Autodesk Inventor part; units mm, degrees
ref_plane "YZ Plane" through (0, 0, 0) normal (1, 0, 0) x (0, 1, 0)
ref_plane "XZ Plane" through (0, 0, 0) normal (0, 1, 0) x (-1, 0, 0)
ref_plane "XY Plane" through (0, 0, 0) normal (0, 0, 1) x (1, 0, 0)
sketch "Battery Flat" plane through (0, 0, 0) normal (0, 0, 1) x (1, 0, 0)
  line L0 (83.566, 88.9) -> (-83.566, 88.9) construction
  line L1 (-83.566, 88.9) -> (-83.566, -88.9) construction
  line L2 (-83.566, -88.9) -> (83.566, -88.9) construction
  line L3 (83.566, -88.9) -> (83.566, 88.9) construction
  line L4 (83.566, 88.9) -> (-83.566, -88.9) construction
  line L5 (-83.566, 88.9) -> (83.566, -88.9) construction
  line L6 (83.566, -88.9) -> (-83.566, -88.9) construction
  line L7 (-83.566, -88.9) -> (-83.566, 88.9) construction
  line L8 (-83.566, 88.9) -> (83.566, 88.9) construction
  line L9 (83.566, 88.9) -> (83.566, -88.9) construction
  point P0 (0, 0)
  dimension "d39" = 167.132
  dimension "d40" = 177.8
sketch "Circuit Breaker" plane through (0, 0, 0) normal (0, 0, 1) x (1, 0, 0)
  line L0 (4.1103, 47.4016) -> (-23.8297, 47.4016) construction
  line L1 (-23.8297, 47.4016) -> (-23.8297, -9.7484) construction
  line L2 (-23.8297, -9.7484) -> (4.1103, -9.7484) construction
  line L3 (4.1103, -9.7484) -> (4.1103, 47.4016) construction
  line L4 (4.1103, 47.4016) -> (-23.8297, -9.7484) construction
  line L5 (-23.8297, 47.4016) -> (4.1103, -9.7484) construction
  circle A0 centre (-23.8297, -9.7484) radius 3.429
  circle A1 centre (4.1103, 47.4016) radius 3.429
  line L6 (4.1103, -9.7484) -> (-23.8297, -9.7484) construction
  line L7 (-23.8297, -9.7484) -> (-23.8297, 47.4016) construction
  line L8 (-23.8297, 47.4016) -> (4.1103, 47.4016) construction
  line L9 (4.1103, 47.4016) -> (4.1103, -9.7484) construction
  line L10 (14.2703, 55.6566) -> (-33.9897, 55.6566) construction
  line L11 (-33.9897, 55.6566) -> (-33.9897, -18.0034) construction
  line L12 (-33.9897, -18.0034) -> (14.2703, -18.0034) construction
  line L13 (14.2703, -18.0034) -> (14.2703, 55.6566) construction
  line L14 (14.2703, 55.6566) -> (-33.9897, -18.0034) construction
  line L15 (-33.9897, 55.6566) -> (14.2703, -18.0034) construction
  point P0 (0, 0)
  point P1 (-9.8597, 18.8266)
  dimension "d62" = 27.94
  dimension "d63" = 57.15
  dimension "d64" = 6.858
  dimension "d65" = 6.858
  dimension "d66" = 48.26
  dimension "d67" = 73.66
sketch "Sketch1" plane through (0, 0, 0) normal (0, 1, 0) x (-1, 0, 0)
  line L0 (95.25, -95.25) -> (-95.25, -95.25) construction
  line L1 (95.25, -90.4875) -> (-95.25, -90.4875)
  line L2 (-95.25, -100.0125) -> (95.25, -100.0125)
  arc A0 (95.25, -100.0125) -> (95.25, -90.4875) centre (95.25, -95.25) ccw
  arc A1 (-95.25, -90.4875) -> (-95.25, -100.0125) centre (-95.25, -95.25) ccw
  line L3 (95.25, 95.25) -> (-95.25, 95.25) construction
  line L4 (95.25, 100.0125) -> (-95.25, 100.0125)
  line L5 (-95.25, 90.4875) -> (95.25, 90.4875)
  arc A2 (95.25, 90.4875) -> (95.25, 100.0125) centre (95.25, 95.25) ccw
  arc A3 (-95.25, 100.0125) -> (-95.25, 90.4875) centre (-95.25, 95.25) ccw
  line L6 (95.25, -95.25) -> (95.25, 95.25) construction
  line L7 (85.725, -95.25) -> (85.725, 95.25)
  line L8 (104.775, 95.25) -> (104.775, -95.25)
  arc A4 (85.725, -95.25) -> (104.775, -95.25) centre (95.25, -95.25) ccw
  arc A5 (104.775, 95.25) -> (85.725, 95.25) centre (95.25, 95.25) ccw
  line L9 (-95.25, -95.25) -> (-95.25, 95.25) construction
  line L10 (-85.725, -95.25) -> (-85.725, 95.25)
  line L11 (-104.775, 95.25) -> (-104.775, -95.25)
  arc A6 (-104.775, -95.25) -> (-85.725, -95.25) centre (-95.25, -95.25) ccw
  arc A7 (-85.725, 95.25) -> (-104.775, 95.25) centre (-95.25, 95.25) ccw
  circle A8 centre (95.25, -95.25) radius 2.4892
  circle A9 centre (95.25, 95.25) radius 2.4892
  circle A10 centre (57.15, -95.25) radius 2.4892
  circle A11 centre (57.15, 95.25) radius 2.4892
  circle A12 centre (19.05, -95.25) radius 2.4892
  circle A13 centre (19.05, 95.25) radius 2.4892
  circle A14 centre (-19.05, -95.25) radius 2.4892
  circle A15 centre (-19.05, 95.25) radius 2.4892
  circle A16 centre (-57.15, -95.25) radius 2.4892
  circle A17 centre (-57.15, 95.25) radius 2.4892
  circle A18 centre (-95.25, -95.25) radius 2.4892
  circle A19 centre (-95.25, 95.25) radius 2.4892
  circle A20 centre (95.25, 57.15) radius 2.4892
  circle A21 centre (-95.25, 57.15) radius 2.4892
  circle A22 centre (95.25, 19.05) radius 2.4892
  circle A23 centre (-95.25, 19.05) radius 2.4892
  circle A24 centre (95.25, -19.05) radius 2.4892
  circle A25 centre (-95.25, -19.05) radius 2.4892
  circle A26 centre (95.25, -57.15) radius 2.4892
  circle A27 centre (-95.25, -57.15) radius 2.4892
  line L12 (-3.175, 100.0125) -> (-3.175, 150.8125)
  line L13 (-3.175, 150.8125) -> (-79.375, 150.8125)
  line L14 (-79.375, 150.8125) -> (-79.375, 100.0125)
  point P0 (0, 0)
  point P1 (0, 0)
  point P2 (0, -95.25)
  point P3 (0, 95.25)
  point P4 (95.25, 0)
  point P5 (-95.25, 0)
  point P6 (0, 0)
  point P7 (0, 0)
  point P8 (85.725, -90.4875)
  point P9 (-85.725, -90.4875)
  point P10 (-85.725, 90.4875)
  point P11 (85.725, 90.4875)
  point P12 (87.0011, -100.0125)
  point P13 (87.0011, 100.0125)
  point P14 (-87.0011, 100.0125)
  point P15 (-87.0011, -100.0125)
  point P16 (-41.275, 150.8125)
  point P17 (-41.275, 150.8125)
  point P18 (-41.275, 125.4125)
  point P19 (-41.275, 125.4125)
  point P20 (-3.175, 125.4125)
  point P21 (-41.275, 125.4125)
  dimension "d41" = 190.5
  dimension "d42" = 190.5
  dimension "d43" = 9.525
  dimension "d44" = 19.05
  dimension "d45" = 4.9784
  dimension "d48" = 38.1
  dimension "d55" = 38.1
  dimension "d60" = 38.1
  dimension "d68" = 76.2
  dimension "d69" = 50.8
  dimension "d75" = 25.4
extrude "Extrusion1" add sketch "Sketch1" along normal blind 6.35 contours A0 L2 A4 L7 L1 | L1 L7 L5 A2 L4 A5 L8 A4 L2 A0 | L7 A4 L2 A6 L10 L1 | L10 A6 L2 A1 L1 | L1 A1 L2 A6 L11 A7 L4 A3 L5 L10 | L7 A5 L4 A2 L5 | L5 L10 A7 L4 A5 L7 | L5 A3 L4 A7 L10
fillet "Fillet1" radius 50.8 4 edges at (87.0011, 3.175, 100.0125) (-87.0011, 3.175, 100.0125) (-87.0011, 3.175, -100.0125) (87.0011, 3.175, -100.0125)
fillet "Fillet1" radius 3.175 4 edges at (-85.725, 3.175, -90.4875) (85.725, 3.175, -90.4875) (85.725, 3.175, 90.4875) (-85.725, 3.175, 90.4875)
extrude "Extrusion2" [suppressed]
fillet "Fillet2" [suppressed]
sketch "Sketch2" plane through (0, 6.35, 0) normal (0, 1, 0) x (1, 0, 0)
  arc A0 (91.5406, -104.023) -> (71.7571, -100.0125) centre (71.7571, -150.8125) ccw
  arc A1 (91.5406, -104.023) -> (104.775, -95.25) centre (95.25, -95.25) ccw
  line L0 (104.775, -95.25) -> (104.775, 95.25)
  arc A2 (104.775, 95.25) -> (91.5406, 104.023) centre (95.25, 95.25) ccw
  arc A3 (71.7571, 100.0125) -> (91.5406, 104.023) centre (71.7571, 150.8125) ccw
  line L1 (71.7571, 100.0125) -> (-71.7571, 100.0125)
  arc A4 (-91.5406, 104.023) -> (-71.7571, 100.0125) centre (-71.7571, 150.8125) ccw
  arc A5 (-91.5406, 104.023) -> (-104.775, 95.25) centre (-95.25, 95.25) ccw
  line L2 (-104.775, 95.25) -> (-104.775, -95.25)
  arc A6 (-104.775, -95.25) -> (-91.5406, -104.023) centre (-95.25, -95.25) ccw
  arc A7 (-71.7571, -100.0125) -> (-91.5406, -104.023) centre (-71.7571, -150.8125) ccw
  line L3 (-71.7571, -100.0125) -> (71.7571, -100.0125)
  circle A8 centre (-95.25, 95.25) radius 2.4892
  circle A9 centre (-57.15, 95.25) radius 2.4892
  circle A10 centre (-19.05, 95.25) radius 2.4892
  circle A11 centre (19.05, 95.25) radius 2.4892
  circle A12 centre (57.15, 95.25) radius 2.4892
  circle A13 centre (95.25, 95.25) radius 2.4892
  circle A14 centre (-95.25, 57.15) radius 2.4892
  circle A15 centre (-95.25, 19.05) radius 2.4892
  circle A16 centre (-95.25, -19.05) radius 2.4892
  circle A17 centre (-95.25, -57.15) radius 2.4892
  circle A18 centre (-95.25, -95.25) radius 2.4892
  circle A19 centre (-57.15, -95.25) radius 2.4892
  circle A20 centre (-19.05, -95.25) radius 2.4892
  circle A21 centre (19.05, -95.25) radius 2.4892
  circle A22 centre (57.15, -95.25) radius 2.4892
  circle A23 centre (95.25, -95.25) radius 2.4892
  circle A24 centre (95.25, 57.15) radius 2.4892
  circle A25 centre (95.25, -57.15) radius 2.4892
  circle A26 centre (95.25, -19.05) radius 2.4892
  circle A27 centre (95.25, 19.05) radius 2.4892
  line L4 (-82.55, 90.4875) -> (82.55, 90.4875)
  arc A28 (85.725, 87.3125) -> (82.55, 90.4875) centre (82.55, 87.3125) ccw
  line L5 (85.725, 87.3125) -> (85.725, -87.3125)
  arc A29 (82.55, -90.4875) -> (85.725, -87.3125) centre (82.55, -87.3125) ccw
  line L6 (82.55, -90.4875) -> (-82.55, -90.4875)
  arc A30 (-85.725, -87.3125) -> (-82.55, -90.4875) centre (-82.55, -87.3125) ccw
  line L7 (-85.725, -87.3125) -> (-85.725, 87.3125)
  arc A31 (-82.55, 90.4875) -> (-85.725, 87.3125) centre (-82.55, 87.3125) ccw
  arc A32 (7.9375, -144.4625) -> (9.525, -146.05) centre (9.525, -144.4625) ccw
  line L8 (7.9375, -144.4625) -> (7.9375, -106.3625)
  arc A33 (7.9375, -106.3625) -> (-3.175, -95.25) centre (-3.175, -106.3625) ccw
  line L9 (-3.175, -95.25) -> (-71.7571, -95.25)
  arc A34 (-71.7571, -95.25) -> (-93.3953, -99.6365) centre (-71.7571, -150.8125) ccw
  arc A35 (-100.0125, -95.25) -> (-93.3953, -99.6365) centre (-95.25, -95.25) ccw
  line L10 (-100.0125, -95.25) -> (-100.0125, 95.25)
  arc A36 (-93.3953, 99.6365) -> (-100.0125, 95.25) centre (-95.25, 95.25) ccw
  arc A37 (-93.3953, 99.6365) -> (-71.7571, 95.25) centre (-71.7571, 150.8125) ccw
  line L11 (-71.7571, 95.25) -> (71.7571, 95.25)
  arc A38 (71.7571, 95.25) -> (93.3953, 99.6365) centre (71.7571, 150.8125) ccw
  arc A39 (100.0125, 95.25) -> (93.3953, 99.6365) centre (95.25, 95.25) ccw
  line L12 (100.0125, 95.25) -> (100.0125, -95.25)
  arc A40 (93.3953, -99.6365) -> (100.0125, -95.25) centre (95.25, -95.25) ccw
  arc A41 (93.3953, -99.6365) -> (89.217, -98.0646) centre (71.7571, -150.8125) ccw
  arc A42 (89.217, -98.0646) -> (74.6125, -108.6141) centre (85.725, -108.6141) ccw
  line L13 (74.6125, -108.6141) -> (74.6125, -144.4625)
  arc A43 (73.025, -146.05) -> (74.6125, -144.4625) centre (73.025, -144.4625) ccw
  line L14 (73.025, -146.05) -> (9.525, -146.05)
  arc A44 (3.175, -106.3625) -> (-3.175, -100.0125) centre (-3.175, -106.3625) ccw
  line L15 (-3.175, -100.0125) -> (78.6894, -100.0125)
  line L16 (-3.175, -104.775) -> (78.6894, -104.775)
  circle A45 centre (12.7, -111.4425) radius 7.9375
  circle A46 centre (69.85, -139.3825) radius 7.9375
  line L17 (12.7, -111.4425) -> (69.85, -139.3825) construction
  line L18 (11.6541, -113.5818) -> (68.8041, -141.5218)
  line L19 (70.8959, -137.2432) -> (13.7459, -109.3032)
  arc A47 (13.7459, -109.3032) -> (11.6541, -113.5818) centre (12.7, -111.4425) ccw
  arc A48 (68.8041, -141.5218) -> (70.8959, -137.2432) centre (69.85, -139.3825) ccw
  line L20 (2.8572, -144.1945) -> (79.6928, -106.6305) construction
  line L21 (3.9031, -146.3338) -> (80.7387, -108.7697)
  line L22 (78.6469, -104.4912) -> (1.8113, -142.0553)
  arc A49 (1.8113, -142.0553) -> (3.9031, -146.3338) centre (2.8572, -144.1945) ccw
  arc A50 (80.7387, -108.7697) -> (78.6469, -104.4912) centre (79.6928, -106.6305) ccw
  line L23 (41.275, -125.4125) -> (41.275, -104.775) construction
  point P0 (0, 0)
  point P1 (74.6125, -111.7648)
  point P2 (46.6967, -125.4125)
  point P3 (64.0934, -133.9176)
  point P4 (74.6125, -133.0325)
  point P5 (41.275, -122.7619)
  point P6 (74.8457, -106.3496)
  point P7 (75.2967, -104.775)
  point P8 (17.0068, -104.775)
  point P9 (20.5483, -112.6289)
  point P10 (7.9375, -139.0602)
  point P11 (35.8533, -125.4125)
  point P12 (18.4566, -116.9074)
  point P13 (7.9375, -117.7925)
  point P14 (65.5432, -146.05)
  point P15 (62.0017, -138.1961)
  point P16 (41.275, -128.0631)
  point P17 (7.9375, -144.3614)
  dimension "d77" = 4.7625
  dimension "d78" = 15.875
  dimension "d79" = 4.7625
  dimension "d80" = 4.7625
extrude "Extrusion3" [suppressed]
fillet "Fillet3" [suppressed]
equation "\"d42\" = d41"
properties part number "7525-18-800-002 Battery Mount" material "Aluminum 6061"
The model under review builds one solid part; all positions refer to its coordinate system, in mm. A direction names the side the tool comes from. Round coordinates to 2 decimals unless told otherwise and drop trailing zeros. Loops run counter-clockwise (first coordinate to the right, second up) from the corner with the lowest first, then second, coordinate; pieces in that order, holes last. Notation, with made-up numbers: (65, 13) - (97, 13) arc R18 cw to (97, 48) - close; hole circle Ø9 at (44, 31.5). An arc over 180 degrees is marked (long way). Write each question's results on one line, items separated by ' | '. Start each with the question number.
Q1. Take a section at B-B on x = 64.5. Give the boundary of the cut face in (y, z), plus the area to 3 significant figures.
Q2. Tool access review of faces 1 (the cylindrical face through (-81.711, 3.219, 100.997)), 2 (the flat face through (-1, 3, -90.488)), 3 (the cylindrical face through (-100.622, 3.131, -103.116)): name each direction out of +Z, -Z, +X, -X, +Y, -Y from which nothing blocks a thin tool from reaching the whole face with its end or side.
Q3. Insertion check: P1, Ø3, axis at x = -95.25, z = -95.25, coming from the -Y side. The pin has a flat end and moves straight along its axis. Give the tip position at first contact, or say it passes through.
Q4. Take a section at C-C on z = 79. Give the boundary of the cut face in (x, y) (3 decimals).
Q5. Wall thickness on line 1 along X through (y, z) = (2, -57) (3 decimals); line 2 along Z through (x, y) = (-19.05, 5.25); line 3 along Z through (x, y) = (44, 1.5): over which ranges is each line inside the solid? List them lowest first. Write a range as [from, to].
Q6. Take a section at A-A on x = -57.15. Give the boundary of the cut face in (y, z).
Q7. Draft analysis for pull direction X (two halves, no side actions). For faces 4 (the flat face through (-104.775, 3, 1)), 5 (the flat face through (1, 0, -92)), 6 (the flat face through (1, 3, -100.012)), 7 (the cylindrical face through (-97.55, 3.13, 58.1)), state which applies: pulls with the +X half, pulls with the -X half, needs draft (parallel to the pull), parting line crosses it, or undercut.
Q8. Take a section at D-D on x = 95.25. Give the boundary of the cut face in (y, z) (3 decimals).
Data:
1) outline: (0, -100.01) - (6.35, -100.01) - (6.35, -90.49) - (0, -90.49) - close; (0, 90.49) - (6.35, 90.49) - (6.35, 100.01) - (0, 100.01) - close | area: 121 mm²
2) face 1: +Z, +Y, -Y | face 2: +Y, -Y | face 3: -Z, +Y, -Y
3) P1: passes through
4) outline: (-104.775, 0) - (-85.725, 0) - (-85.725, 6.35) - (-104.775, 6.35) - close; (85.725, 0) - (104.775, 0) - (104.775, 6.35) - (85.725, 6.35) - close
5) line 1: x = [-104.775, -97.735], [-92.765, -85.725], [85.725, 92.765], [97.735, 104.775] | line 2: z = [-100.01, -97.74], [-92.76, -90.49], [90.49, 92.76], [97.74, 100.01] | line 3: z = [-100.01, -90.49], [90.49, 100.01]
6) outline: (0, -100.01) - (6.35, -100.01) - (6.35, -97.74) - (0, -97.74) - close; (0, -92.76) - (6.35, -92.76) - (6.35, -90.49) - (0, -90.49) - close; (0, 90.49) - (6.35, 90.49) - (6.35, 92.76) - (0, 92.76) - close; (0, 97.74) - (6.35, 97.74) - (6.35, 100.01) - (0, 100.01) - close
7) face 4: pulls with the -X half | face 5: needs draft | face 6: undercut | face 7: undercut
8) outline: (0, -104.775) - (6.35, -104.775) - (6.35, -97.739) - (0, -97.739) - close; (0, -92.761) - (6.35, -92.761) - (6.35, -59.639) - (0, -59.639) - close; (0, -54.661) - (6.35, -54.661) - (6.35, -21.539) - (0, -21.539) - close; (0, -16.561) - (6.35, -16.561) - (6.35, 16.561) - (0, 16.561) - close; (0, 21.539) - (6.35, 21.539) - (6.35, 54.661) - (0, 54.661) - close; (0, 59.639) - (6.35, 59.639) - (6.35, 92.761) - (0, 92.761) - close; (0, 97.739) - (6.35, 97.739) - (6.35, 104.775) - (0, 104.775) - close
